Autodesk Inventor part; units mm, degrees
ref_plane "YZ Plane" through (0, 0, 0) normal (1, 0, 0) x (0, 1, 0)
ref_plane "XZ Plane" through (0, 0, 0) normal (0, 1, 0) x (-1, 0, 0)
ref_plane "XY Plane" through (0, 0, 0) normal (0, 0, 1) x (1, 0, 0)
sketch "スケッチ1" plane through (0, 0, 0) normal (0, 0, 1) x (1, 0, 0)
  line L0 (0, 0) -> (7, 0)
  line L1 (7, 0) -> (7, 40)
  line L2 (7, 40) -> (0, 40)
  line L3 (0, 40) -> (0, 0)
  dimension "d0" = 7
  dimension "d1" = 40
extrude "押し出し1" add sketch "スケッチ1" along normal blind 2
sketch "スケッチ2" plane through (0, 0, 2) normal (0, 0, 1) x (1, 0, 0)
  line L0 (7, 0) -> (7, 40)
  line L1 (7, 40) -> (0, 40)
  line L2 (0, 0) -> (7, 0)
  point P0 (3.5, 35)
  point P1 (3.5, 5)
  dimension "d4" = 3.5
  dimension "d5" = 5
  dimension "d6" = 3.5
  dimension "d7" = 5
hole "穴1" at (3.5, 35, 2) at (3.5, 5, 2) direction (0, 0, -1) diameter 3.2 end through all
sketch "スケッチ3" plane through (0, 0, 2) normal (0, 0, 1) x (1, 0, 0)
  point P0 (0, 0)
properties part number "リンク40×7×2"
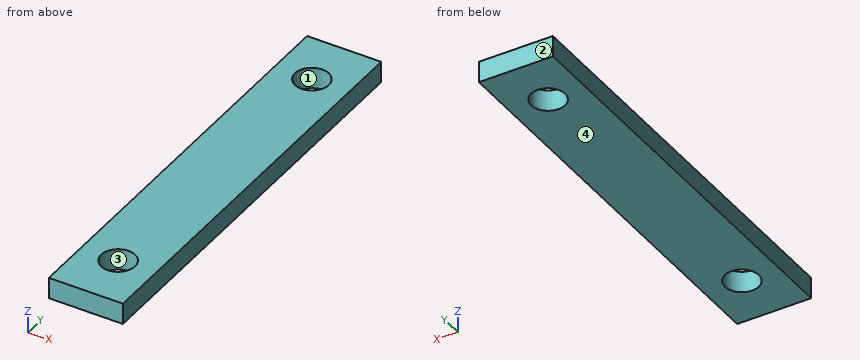
Build history of the part. All positions in model axes, mm. Face numbers are marked on the shaded views. Round coordinates to 2 decimals unless told otherwise and drop trailing zeros. Order: outer loops, then holes, each group sorted by start corner. A loop starts at its lowest first (then second) coordinate and runs counter-clockwise, first axis right, second up. Notation, with made-up numbers: (61, -36.5) -> (110, -36.5) arc R32 ccw to (110, -10.5) -> close; hole circle Ø11 at (69.25, 10). An arc over 180 degrees is marked (long way). Answer in a Markdown table with one row per item.
1) Mould opens along Y. For the marked faces 1, 2, 3 and 4 say: released by +Y, released by -Y, zero draft, split by the parting line, or undercut.
Values:
| item | result |
|---|---|
| face 1 | undercut |
| face 2 | released by +Y |
| face 3 | undercut |
| face 4 | zero draft |
2) Band-saw the part on D-D on y = 34.5. Give the cut face in (x, z), and give its area (3 significant figures).
Values:
| item | result |
|---|---|
| outline | (0, 0) -> (1.98, 0) -> (1.98, 2) -> (0, 2) -> close; (5.02, 0) -> (7, 0) -> (7, 2) -> (5.02, 2) -> close |
| area | 7.92 mm2 |
3) Wall check: L1, parallel to Y at x = 3.5, z = 0.7; L2, parallel to X at y = 5, z = 1.4; L3, parallel to Y at x = 2.25, z = 0.7. Give the ranges that are in metal, low to high.
Values:
| item | result |
|---|---|
| L1 | 0 to 3.4, 6.6 to 33.4, 36.6 to 40 |
| L2 | 0 to 1.9, 5.1 to 7 |
| L3 | 0 to 4, 6 to 34, 36 to 40 |
4) Pin check, flat tips, straight feed: P1, Ø2.5, axis at x = 3.5, y = 35, coming from the -Z side; P2, Ø4, axis at x = 1.5, y = 12, coming from the -Z side. Stop position of each tip, or through.
Values:
| item | result |
|---|---|
| P1 | through |
| P2 | z = 0 |
5) Band-saw the part on C-C on z = 0.5. Give the cut face in (x, y).
Values:
| item | result |
|---|---|
| outline | (0, 0) -> (7, 0) -> (7, 40) -> (0, 40) -> close; hole circle Ø3.2 at (3.5, 5); hole circle Ø3.2 at (3.5, 35) |
6) Band-saw the part on A-A on x = 3.5. Give the cut face in (y, z).
Values:
| item | result |
|---|---|
| outline | (0, 0) -> (3.4, 0) -> (3.4, 2) -> (0, 2) -> close; (6.6, 0) -> (33.4, 0) -> (33.4, 2) -> (6.6, 2) -> close; (36.6, 0) -> (40, 0) -> (40, 2) -> (36.6, 2) -> close |
7) Band-saw the part on B-B on y = 5. Give the cut face in (x, z), and give its area (3 significant figures).
Values:
| item | result |
|---|---|
| outline | (0, 0) -> (1.9, 0) -> (1.9, 2) -> (0, 2) -> close; (5.1, 0) -> (7, 0) -> (7, 2) -> (5.1, 2) -> close |
| area | 7.60 mm2 |
